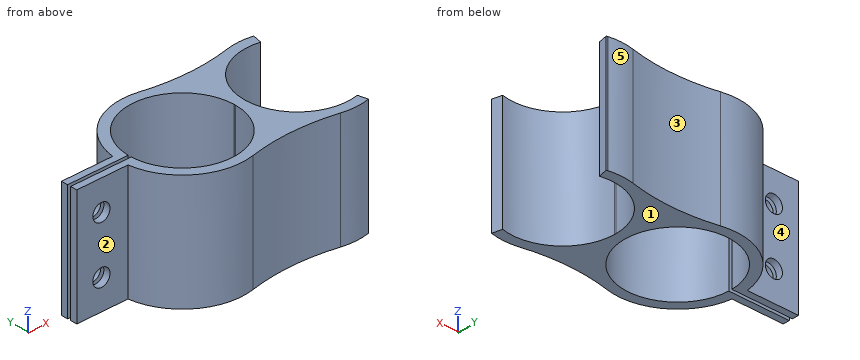
```python
from build123d import *

# Parameters (mm, degrees)
F1_DEPTH = 35
F3_DEPTH = 40
F4_DEPTH = 35
F5_R     = 2.6
F6_DEPTH = 12.5


with BuildPart() as f1:
    # F0 (on Top) → F1 (new body)
    with BuildSketch(Plane.XY):
        with BuildLine():
            ThreePointArc((30.7878121478, 18.5280684134), (17.4981090624, 17.03775814), (4.208405977, 18.5280684134))
            ThreePointArc((4.208405977, 18.5280684134), (-19, 0), (4.208405977, -18.5280684134))
            ThreePointArc((4.208405977, -18.5280684134), (17.4981090624, -17.03775814), (30.7878121478, -18.5280684134))
            ThreePointArc((30.7878121478, -18.5280684134), (35.0954185177, -18.999741032), (39.3978648328, -18.4831140844))
            Line((39.3978648328, -18.4831140844), (38.7028679842, -15.5647276501))
            ThreePointArc((38.7028679842, -15.5647276501), (25.1801121151, -12.6350331541), (18.9982711603, -0.2563062995))
            ThreePointArc((18.9982711603, -0.2563062995), (18.9962181249, 0), (18.9982711603, 0.2563062995))
            ThreePointArc((18.9982711603, 0.2563062995), (25.0510572832, 12.5337055907), (38.3828757407, 15.6374726281))
            Line((38.3828757407, 15.6374726281), (39.0178740437, 18.5694987458))
            ThreePointArc((39.0178740437, 18.5694987458), (38.8268942308, 18.6098339748), (38.6355101254, 18.6482051076))
            ThreePointArc((38.6355101254, 18.6482051076), (38.6103354346, 18.6531004412), (38.585154159, 18.6579617896))
            ThreePointArc((38.585154159, 18.6579617896), (34.6797472339, 18.9973641902), (30.7878121478, 18.5280684134))
        make_face()
        with BuildLine():
            ThreePointArc((15.9979469646, 0.2563062995), (15.9994867329, 0.1281572609), (16, 0))
            ThreePointArc((16, 0), (15.9994867329, -0.1281572609), (15.9979469646, -0.2563062995))
            ThreePointArc((15.9979469646, -0.2563062995), (-16, 0), (15.9979469646, 0.2563062995))
        make_face(mode=Mode.SUBTRACT)
    extrude(amount=F1_DEPTH)

    # F2 (on Top) → F3 (cut)
    with BuildSketch(Plane.XY):
        Polygon((-18.4108596295, -0.5), (-14.4108596295, -0.5), (-14.4108596295, 0.5), (-18.4108596295, 0.5), (-22.4108596295, 0.5), (-22.4108596295, -0.5), align=None)
    extrude(amount=F3_DEPTH, mode=Mode.SUBTRACT)

    # F2 (on Top) → F4 (join)
    with BuildSketch(Plane.XY):
        Polygon((-22.4108596295, 0.5), (-18.4108596295, 0.5), (-18.4108596295, 2.5), (-34.4108596295, 2.5), (-34.4108596295, 0.5), align=None)
        Polygon((-18.4108596295, -2.5), (-18.4108596295, -0.5), (-22.4108596295, -0.5), (-34.4108596295, -0.5), (-34.4108596295, -2.5), align=None)
    extrude(amount=F4_DEPTH)

    # F5 (on Front) → F6 (cut, symmetric)
    with BuildSketch(Plane.XZ):
        with Locations((-26.9108596295, 26)):
            Circle(F5_R)
        with Locations((-26.9108596295, 9)):
            Circle(F5_R)
    extrude(amount=F6_DEPTH, both=True, mode=Mode.SUBTRACT)


solid = f1.part
```
Part model, mm, in its own coordinate system. Face numbers are marked on the shaded views. A direction names the side the tool comes from. Round coordinates to 2 decimals unless told otherwise and drop trailing zeros. Write each loop counter-clockwise with the first axis right and the second up, starting at its lowest first coordinate (ties: lowest second). Pieces come first, ordered by that corner, then holes. Notation, with made-up numbers: (2.25, 65.25) -> (38.25, 65.25) arc R7 cw to (38.25, 71.25) -> close; hole circle Ø11 at (15, 9). An arc over 180 degrees is marked (long way). Return JSON: item names as keys, results as strings. Group by question number.
Q1. Saw through at D-D on x = -27. Write the cut outline in (y, z).
Q2. Which spindle directions (+Z, -Z, +X, -X, +Y, -Y) get a long thin tool onto all of the face, cutting with end or side? Do the marked faces 1 and 2. Say none if no direction does.
Q3. Pin check, flat tips, straight feed: pin 1 (12 mm diameter, centred on x = -14, z = 23.5, fed in from -Y); pin 2 (1.5 mm diameter, centred on y = -13, z = 4.5, fed in from -X); pin 3 (5 mm diameter, centred on y = 9, z = 6.5, fed in from -X). Stop position of each tip, or through.
Q4. Saw through at A-A on z = 9. Write the cut outline in (x, y).
Q5. Saw through at B-B on x = 0. Write the cut outline in (y, z).
Q6. Saw through at C-C on z = 31. Write the cut outline in (x, y).
Q7. Mould opens along X. For the marked faces 3, 4 and 5 say: pulls with the +X half, pulls with the -X half, needs draft (parallel to the pull), parting line crosses it, or undercut.
Q8. Probe L1, parallel to Y at x = 34.5, z = 10; L2, parallel to X at y = -1.4, z = 26; L3, parallel to X at y = 2, z = 7. List the from-to ranges inside material, lowest first. Write a range as [from, to].
Answer:
{
 "1": {"outline": "(-2.5, 0) -> (-0.5, 0) -> (-0.5, 6.4) -> (-2.5, 6.4) -> close; (-2.5, 11.6) -> (-0.5, 11.6) -> (-0.5, 23.4) -> (-2.5, 23.4) -> close; (-2.5, 28.6) -> (-0.5, 28.6) -> (-0.5, 35) -> (-2.5, 35) -> close; (0.5, 0) -> (2.5, 0) -> (2.5, 6.4) -> (0.5, 6.4) -> close; (0.5, 11.6) -> (2.5, 11.6) -> (2.5, 23.4) -> (0.5, 23.4) -> close; (0.5, 28.6) -> (2.5, 28.6) -> (2.5, 35) -> (0.5, 35) -> close"},
 "2": {"face 1": "-Z, +X, -X, +Y, -Y", "face 2": "+Z, -Z, -X, -Y"},
 "3": {"pin 1": "y = -17.23", "pin 2": "x = -14.52", "pin 3": "x = -17.85"},
 "4": {"outline": "(-34.41, -2.5) -> (-29.51, -2.5) -> (-29.51, -0.5) -> (-34.41, -0.5) -> close; (-34.41, 0.5) -> (-29.51, 0.5) -> (-29.51, 2.5) -> (-34.41, 2.5) -> close; (-24.31, -2.5) -> (-18.83, -2.5) arc R19 ccw to (4.21, -18.53) arc R60 cw to (30.79, -18.53) arc R19 ccw to (39.4, -18.48) -> (38.7, -15.56) arc R16 cw (long way) to (38.38, 15.64) -> (39.02, 18.57) arc R19 ccw to (38.64, 18.65) arc R19 ccw to (38.59, 18.66) arc R19 ccw to (30.79, 18.53) arc R60 cw to (4.21, 18.53) arc R19 ccw to (-18.83, 2.5) -> (-24.31, 2.5) -> (-24.31, 0.5) -> (-15.99, 0.5) arc R16 cw (long way) to (-15.99, -0.5) -> (-24.31, -0.5) -> close"},
 "5": {"outline": "(-19, 0) -> (-16, 0) -> (-16, 35) -> (-19, 35) -> close; (16, 0) -> (19, 0) -> (19, 35) -> (16, 35) -> close"},
 "6": {"outline": "(-34.41, -2.5) -> (-18.83, -2.5) arc R19 ccw to (4.21, -18.53) arc R60 cw to (30.79, -18.53) arc R19 ccw to (39.4, -18.48) -> (38.7, -15.56) arc R16 cw (long way) to (38.38, 15.64) -> (39.02, 18.57) arc R19 ccw to (38.64, 18.65) arc R19 ccw to (38.59, 18.66) arc R19 ccw to (30.79, 18.53) arc R60 cw to (4.21, 18.53) arc R19 ccw to (-18.83, 2.5) -> (-34.41, 2.5) -> (-34.41, 0.5) -> (-15.99, 0.5) arc R16 cw (long way) to (-15.99, -0.5) -> (-34.41, -0.5) -> close"},
 "7": {"face 3": "undercut", "face 4": "needs draft", "face 5": "undercut"},
 "8": {"L1": "[-18.99, -15.99], [15.99, 18.99]", "L2": "[-34.41, -29.51], [-24.31, -15.94], [15.94, 19.06]", "L3": "[-34.41, -28.57], [-25.25, -15.87], [15.87, 19.12]"}
}
